Read the model definition and answer for the solid it produces. Units are mm, in the model's axes. A direction names the side the tool comes from. Coordinates: 2 decimals unless noted, no trailing zeros. Write each loop counter-clockwise with the first axis right and the second up, starting at its lowest first coordinate (ties: lowest second). Pieces come first, ordered by that corner, then holes.
1) The part is cut by section A-A (x = 42). Determine the outline of the cut face in (y, z).
2) Each of these flat-tipped pins is pushed along its axis until it touches: pin 1 Ø1.6 at (x, y) = (-27.25, 59.02) entering from -Z; pin 2 Ø2 at (y, z) = (49, 15) entering from -X; pin 3 Ø3 at (x, y) = (-31.5, 40) entering from -Z; pin 4 Ø7.5 at (y, z) = (80, 11) entering from +X. Where does it stop, or does it pass through?
3) Determine the mould class of faces 1 (the face through (-29.51, 17.6, 8.87)), 2 (the face through (-30, 13, 0)) for opening direction X: +X half, -X half, draft (parallel to the pull), parting line (faces both ways), or undercut.
4) Find the intervals of material crossed by line 1 (X direction, y = 54, z = 11); line 2 (X direction, y = -15, z = 19.75); line 3 (Y direction, x = -34.5, z = 2.5), in increasing order.
5) Which of the six approach directions +Z, -Z, +X, -X, +Y, -Y give full straight-line access (tool end or side, diameter ignored) to faces 3 (the face through (2, 65, 6)), 4 (the face through (-75.61, -43.46, 22.48)), 5 (the face through (-8.75, 83, 9)), 6 (the face through (-1, -31.105, 12))?
6) The part is cut by section B-B (y = 44.5). Determine the outline of the cut face in (x, z), then the cut area to 3 significant figures.
7) The part is cut by section C-C (z = 15.75). Give the number of separate pieces and of enclosed holes in the cut face, then the cut area to 3 significant figures.
from build123d import *

# Parameters (mm, degrees)
PAD_DEPTH             = 24
POCKET_DEPTH          = 3
SKETCH002_W           = 70
SKETCH002_H           = 18.5
POCKET001_DEPTH       = 18
POLARPATTERN_COUNT    = 3
POCKET002_DEPTH       = 6
CHAMFER_SIZE          = 8
FILLET_R              = 13
FILLET001_R           = 11
CHAMFER001_SIZE       = 16.1
FILLET002_R           = 11
FILLET003_R           = 12
POCKET003_DEPTH       = 6
POCKET004_DEPTH       = 18
POCKET005_DEPTH       = 21.001
SKETCH007_W           = 15.5
SKETCH007_H           = 15
POCKET006_DEPTH       = 5
SKETCH010_W           = 13.6
SKETCH010_H           = 9
POCKET009_DEPTH       = 15.5
POCKET010_DEPTH       = 3
SKETCH012_R           = 1.85
SKETCH012_R_2         = 0.99
POCKET011_DEPTH       = 498.0492855781
POLARPATTERN001_COUNT = 3
POCKET012_DEPTH       = 12
POCKET013_DEPTH       = 3


with BuildPart() as part:
    # Sketch → Pad (new body)
    with BuildSketch(Plane.XY):
        Polygon((0, 112.2094915052), (-97.1762701892, -56.1047457526), (97.1762701892, -56.1047457526), align=None)
        Polygon((0, 62.2094915052), (-53.875, -31.1047457526), (53.875, -31.1047457526), align=None, mode=Mode.SUBTRACT)
    extrude(amount=PAD_DEPTH)

    # Sketch001 (on Face8 of Pad) → Pocket (cut)
    with BuildSketch(Plane.XY.offset(24)):
        Polygon((0, 98.2094915052), (-85.0519145362, -49.1047457526), (85.0519145362, -49.1047457526), align=None)
        Polygon((0, 76.2094915052), (-65.999355653, -38.1047457526), (65.999355653, -38.1047457526), align=None, mode=Mode.SUBTRACT)
    extrude(amount=-POCKET_DEPTH, mode=Mode.SUBTRACT)

    # Sketch002 (on Face4 of Pocket) → Pocket001 (cut)
    with BuildSketch(Plane(origin=(0, 0, 0), x_dir=(1, 0, 0), z_dir=(0, 0, -1))):
        with Locations((0, 43.6047457526)):
            Rectangle(SKETCH002_W, SKETCH002_H)
    pocket001 = extrude(amount=-POCKET001_DEPTH, mode=Mode.SUBTRACT)

    # PolarPattern: Pocket001 ×3 about axis
    polarpattern_axis = Axis((0, 0, 0), (0, 0, -1))
    for i in range(1, POLARPATTERN_COUNT):
        add(pocket001.rotate(polarpattern_axis, i * 360 / POLARPATTERN_COUNT), mode=Mode.SUBTRACT)

    # Sketch003 (on Face4 of PolarPattern) → Pocket002 (cut)
    with BuildSketch(Plane(origin=(0, 0, 0), x_dir=(1, 0, 0), z_dir=(0, 0, -1))):
        Polygon((0, -100.2094915052), (86.7839653438, 50.1047457526), (-86.7839653438, 50.1047457526), align=None)
        Polygon((0, -74.2094915052), (64.2673048454, 37.1047457526), (-64.2673048454, 37.1047457526), align=None, mode=Mode.SUBTRACT)
    extrude(amount=-POCKET002_DEPTH, mode=Mode.SUBTRACT)

    # Chamfer
    chamfer_edges = [part.edges().sort_by_distance(p)[0] for p in [
        (-53.875, -31.104746, 12),
        (53.875, -31.104746, 12),
        (0, 62.209492, 12),
    ]]
    chamfer(chamfer_edges, length=CHAMFER_SIZE)

    # Fillet
    fillet_edges = [part.edges().sort_by_distance(p)[0] for p in [
        (0, 100.209492, 3),
        (-86.783965, -50.104746, 3),
        (86.783965, -50.104746, 3),
    ]]
    fillet(fillet_edges, radius=FILLET_R)

    # Fillet001
    fillet001_edges = [part.edges().sort_by_distance(p)[0] for p in [
        (0, 74.209492, 3),
        (64.267305, -37.104746, 3),
        (-64.267305, -37.104746, 3),
    ]]
    fillet(fillet001_edges, radius=FILLET001_R)

    # Chamfer001
    chamfer001_edges = [part.edges().sort_by_distance(p)[0] for p in [
        (97.17627, -56.104746, 12),
        (0, 112.209492, 12),
        (-97.17627, -56.104746, 12),
    ]]
    chamfer(chamfer001_edges, length=CHAMFER001_SIZE)

    # Fillet002
    fillet002_edges = [part.edges().sort_by_distance(p)[0] for p in [
        (0, 98.209492, 22.5),
        (-85.051915, -49.104746, 22.5),
        (85.051915, -49.104746, 22.5),
    ]]
    fillet(fillet002_edges, radius=FILLET002_R)

    # Fillet003
    fillet003_edges = [part.edges().sort_by_distance(p)[0] for p in [
        (65.999356, -38.104746, 22.5),
        (0, 76.209492, 22.5),
        (-65.999356, -38.104746, 22.5),
    ]]
    fillet(fillet003_edges, radius=FILLET003_R)

    # Sketch004 (on Face60 of Fillet003) → Pocket003 (cut)
    with BuildSketch(Plane(origin=(0, 0, 6), x_dir=(1, 0, 0), z_dir=(0, 0, -1))):
        Polygon((-8.75, -71.2664825043), (8.75, -71.2664825043), (8.75, -94.7664825043), (4, -94.7664825043), (4, -98.2664825043), (-4, -98.2664825043), (-4, -94.7664825043), (-8.75, -94.7664825043), align=None)
    extrude(amount=-POCKET003_DEPTH, mode=Mode.SUBTRACT)

    # Sketch005 (on Face29 of Pocket003) → Pocket004 (cut)
    with BuildSketch(Plane(origin=(0, 0, 0), x_dir=(1, 0, 0), z_dir=(0, 0, -1))):
        Polygon((46.1715988394, 38.9547457526), (68.6882593378, 51.9547457526), (79.3382593378, 33.508404652), (56.8215988394, 20.508404652), align=None)
    extrude(amount=-POCKET004_DEPTH, mode=Mode.SUBTRACT)

    # Sketch006 (on Face1 of Pocket004) → Pocket005 (cut, through all)
    with BuildSketch(Plane.XY.offset(21)):
        with BuildLine():
            ThreePointArc((1.5, 85.0404521425), (0, 86.5404521425), (-1.5, 85.0404521425))
            Line((-1.5, 85.0404521425), (-1.5, 66.0404521425))
            ThreePointArc((-1.5, 66.0404521425), (0, 64.5404521425), (1.5, 66.0404521425))
            Line((1.5, 85.0404521425), (1.5, 66.0404521425))
        make_face()
    extrude(amount=-POCKET005_DEPTH, mode=Mode.SUBTRACT)

    # Sketch007 (on Face24 of Pocket005) → Pocket006 (cut)
    with BuildSketch(Plane(origin=(-48.5881350946, 28.0523728763, 0), x_dir=(-0.5, -0.8660254038, 0), z_dir=(-0.8660254038, 0.5, 0))):
        with Locations((-47.3262701892, 13.5)):
            Rectangle(SKETCH007_W, SKETCH007_H)
    extrude(amount=-POCKET006_DEPTH, mode=Mode.SUBTRACT)

    # Sketch010 (on Face79 of Pocket006) → Pocket009 (cut)
    with BuildSketch(Plane(origin=(-44.2580080757, 25.5523728763, 0), x_dir=(-0.5, -0.8660254038, 0), z_dir=(-0.8660254038, 0.5, 0))):
        with Locations((-47.3262701892, 13.5)):
            Rectangle(SKETCH010_W, SKETCH010_H)
    extrude(amount=-POCKET009_DEPTH, mode=Mode.SUBTRACT)

    # Sketch011 (on Face21 of Pocket009) → Pocket010 (cut)
    with BuildSketch(Plane(origin=(0, 0, 6), x_dir=(1, 0, 0), z_dir=(0, 0, -1))):
        Polygon((-21.0413798427, -59.7570681827), (-11.6817654684, -54.3532923042), (-6.658482036, -63.0538744299), (-16.0180964103, -68.4576503084), align=None)
    extrude(amount=-POCKET010_DEPTH, mode=Mode.SUBTRACT)

    # Sketch012 (on Face54 of Pocket010) → Pocket011 (cut, through all)
    with BuildSketch(Plane(origin=(0, 0, 0), x_dir=(1, 0, 0), z_dir=(0, 0, -1))):
        with Locations((-13.5, -82.7032108255)):
            Circle(SKETCH012_R)
        with Locations((13.5, -82.7032108255)):
            Circle(SKETCH012_R)
        with Locations((-6.25, -96.5164825043)):
            Circle(SKETCH012_R_2)
        with Locations((6.25, -96.5164825043)):
            Circle(SKETCH012_R_2)
        with Locations((-27.2463245869, -59.0174730012)):
            Circle(SKETCH012_R_2)
        with Locations((-47.1862074814, -27.2405827309)):
            Circle(SKETCH012_R_2)
        with Locations((-64.7337931796, 5.9127272486)):
            Circle(SKETCH012_R_2)
        with Locations((-10.791841915, -49.5174730012)):
            Circle(SKETCH012_R_2)
        with Locations((-28.3394276132, -16.3641630217)):
            Circle(SKETCH012_R_2)
        with Locations((-48.2793105078, 15.4127272487)):
            Circle(SKETCH012_R_2)
    pocket011 = extrude(amount=-POCKET011_DEPTH, mode=Mode.SUBTRACT)

    # PolarPattern001: Pocket011 ×3 about axis
    polarpattern001_axis = Axis((0, 0, 0), (0, 0, -1))
    for i in range(1, POLARPATTERN001_COUNT):
        add(pocket011.rotate(polarpattern001_axis, i * 360 / POLARPATTERN001_COUNT), mode=Mode.SUBTRACT)

    # Sketch013 (on Face132 of PolarPattern001) → Pocket012 (cut)
    with BuildSketch(Plane(origin=(0, 0, 6), x_dir=(1, 0, 0), z_dir=(0, 0, -1))):
        Polygon((58.553649647, 21.508404652), (63.3167893678, 24.258404652), (66.3167893678, 19.0622522293), (61.553649647, 16.3122522293), align=None)
    extrude(amount=-POCKET012_DEPTH, mode=Mode.SUBTRACT)

    # Sketch014 (on Face127 of Pocket012) → Pocket013 (cut)
    with BuildSketch(Plane(origin=(0, 0, 6), x_dir=(1, 0, 0), z_dir=(0, 0, -1))):
        Polygon((-74.3478338252, 33.3748379063), (-65.8478338252, 48.0972697706), (-52.8574527684, 40.5972697706), (-61.3574527684, 25.8748379063), align=None)
    extrude(amount=-POCKET013_DEPTH, mode=Mode.SUBTRACT)


solid = part.part
Reported:
1. outline: (-56.1, 0) - (-50.1, 0) - (-50.1, 6) - (-37.1, 6) - (-37.1, 0) - (-31.1, 0) - (-31.1, 24) - (-38.1, 24) - (-38.1, 21) - (-49.1, 21) - (-49.1, 24) - (-56.1, 24) - close; (-10.54, 0) - (-4.04, 0) - (-4.04, 18) - (32.96, 18) - (32.96, 0) - (39.46, 0) - (39.46, 24) - (25.46, 24) - (25.46, 21) - (3.46, 21) - (3.46, 24) - (-10.54, 24) - close
2. pin 1: passes through
2. pin 2: stops at x = -37.07
2. pin 3: stops at z = 18
2. pin 4: stops at x = 20.76
3. face 1: undercut
3. face 2: draft
4. line 1: x = -33.61 to -29.85, -23.53 to -12.48, -9.94 to -4.74, 4.74 to 23.53, 29.85 to 33.61
4. line 2: x = -73.44 to -49.18, -47.38 to -44.58, 44.58 to 47.38, 49.18 to 73.44
4. line 3: y = -56.1 to -52.85, -34.35 to -31.1, 2.45 to 8.95, 45.95 to 52.45
5. face 3: -Z
5. face 4: +Z
5. face 5: none
5. face 6: +Z, -Z
6. outline: (-39.09, 0) - (-35.34, 0) - (-35.34, 18) - (-13.98, 18) - (-13.98, 0) - (-10.22, 0) - (-10.22, 24) - (-18.31, 24) - (-18.31, 21) - (-31.01, 21) - (-31.01, 24) - (-39.09, 24) - close; (10.22, 0) - (13.98, 0) - (13.98, 18) - (35.34, 18) - (35.34, 0) - (39.09, 0) - (39.09, 24) - (31.01, 24) - (31.01, 21) - (18.31, 21) - (18.31, 24) - (10.22, 24) - close
6. area: 540 mm2
7. separate pieces: 1
7. enclosed holes: 36
7. area: 6,110 mm2
